```python
from build123d import *

# Parameters (mm, degrees)
SKETCH_1_R      = 4
EXTRUDE_2_DEPTH = 3
SKETCH_2_W      = 410
SKETCH_2_H      = 375
SKETCH_2_W_2    = 404
SKETCH_2_H_2    = 369
EXTRUDE_3_DEPTH = 105


with BuildPart() as part:
    # 草圖1 → 填料-伸長2 (new body)
    with BuildSketch(Plane(origin=(0, 0, 0), x_dir=(1, 0, 0), z_dir=(0, 1, 0))):
        Polygon((0, 0), (0, -375), (40, -375), (40, -415), (397, -415), (397, -375), (410, -375), (410, 0), (397, 0), (397, 40), (40, 40), (40, 0), align=None)
        with Locations((159, 20)):
            Circle(SKETCH_1_R, mode=Mode.SUBTRACT)
        with Locations((278, 20)):
            Circle(SKETCH_1_R, mode=Mode.SUBTRACT)
        with Locations((278, -395)):
            Circle(SKETCH_1_R, mode=Mode.SUBTRACT)
        with Locations((159, -395)):
            Circle(SKETCH_1_R, mode=Mode.SUBTRACT)
    extrude(amount=EXTRUDE_2_DEPTH)

    # 草圖2 → 填料-伸長3 (add)
    with BuildSketch(Plane(origin=(0, 3, 0), x_dir=(1, 0, 0), z_dir=(0, 1, 0))):
        with Locations((205, -187.5)):
            Rectangle(SKETCH_2_W, SKETCH_2_H)
        with Locations((205, -187.5)):
            Rectangle(SKETCH_2_W_2, SKETCH_2_H_2, mode=Mode.SUBTRACT)
    extrude(amount=EXTRUDE_3_DEPTH)


solid = part.part
```
CAD build for the part. Positions are in the model's coordinates, mm. A direction names the side the tool comes from. Round coordinates to 2 decimals unless told otherwise and drop trailing zeros. Write each loop counter-clockwise with the first axis right and the second up, starting at its lowest first coordinate (ties: lowest second). Pieces come first, ordered by that corner, then holes. Notation, with made-up numbers: (77, 4.25) - (109, 4.25) arc R22 cw to (109, 12.25) - close; hole circle Ø3 at (42.25, 32). An arc over 180 degrees is marked (long way). Write item = value, one per line. Start each with the question number.
Q1. Drop flat-ended pins along their axis: pin 1 (4 mm diameter, centred on x = 269, z = 293, fed in from +Y); pin 2 (3.5 mm diameter, centred on y = 1.5, z = -11, fed in from +X); pin 3 (3.5 mm diameter, centred on y = 2, z = 392, fed in from -X); pin 4 (5 mm diameter, centred on x = 159, z = -20, fed in from -Y). Give the stop position or say it passes through.
Q2. Probe L1, parallel to Z at x = 278, y = 0.8; L2, parallel to X at y = 0.9, z = -20; L3, parallel to X at y = 42, z = 199.5. List the from-to ranges inside material, lowest first. Write a range as from..to.
Q3. Band-saw the part on A-A (x = 192). Give the cut face in (y, z).
Q4. Mould opens along Z. For faces 1 (the flat face through (0, 53, 190)), 2 (the flat face through (202, 55, 3)) say: pulls with the +Z half, pulls with the -Z half, needs draft (parallel to the pull), parting line crosses it, or undercut.
Q5. Band-saw the part on C-C (z = 152). Give the cut face in (x, y).
Q6. Band-saw the part on B-B (y = 73). Give the cut face in (x, z), then the cut area to 3 significant figures.
Q7. Which spindle directions (+Z, -Z, +X, -X, +Y, -Y) get a long thin tool onto all of the face, cutting with end or side? Do faces 3 (the flat face through (202, 0, 184)), 4 (the flat face through (216, 3, -20)), 5 (the flat face through (216, 3, 395)), 6 (the flat face through (202, 3, 185)), 7 (the flat face through (410, 53, 190)). Say none if no direction does.
Answers below:
q1.pin_1 = 3
q1.pin_2 = 397
q1.pin_3 = 40
q1.pin_4 = through
q2.L1 = -40..-24, -16..391, 399..415
q2.L2 = 40..155, 163..274, 282..397
q2.L3 = 0..3, 407..410
q3.outline = (0, -40) - (3, -40) - (3, 0) - (108, 0) - (108, 3) - (3, 3) - (3, 372) - (108, 372) - (108, 375) - (3, 375) - (3, 415) - (0, 415) - close
q4.face_1 = needs draft
q4.face_2 = undercut
q5.outline = (0, 0) - (410, 0) - (410, 108) - (407, 108) - (407, 3) - (3, 3) - (3, 108) - (0, 108) - close
q6.outline = (0, 0) - (410, 0) - (410, 375) - (0, 375) - close; hole (3, 3) - (407, 3) - (407, 372) - (3, 372) - close
q6.area = 4,670 mm2
q7.face_3 = +Z, -Z, +X, -X, -Y
q7.face_4 = -Z, +X, -X, +Y
q7.face_5 = +Z, +X, -X, +Y
q7.face_6 = +Y
q7.face_7 = +Z, -Z, +X, +Y, -Y
